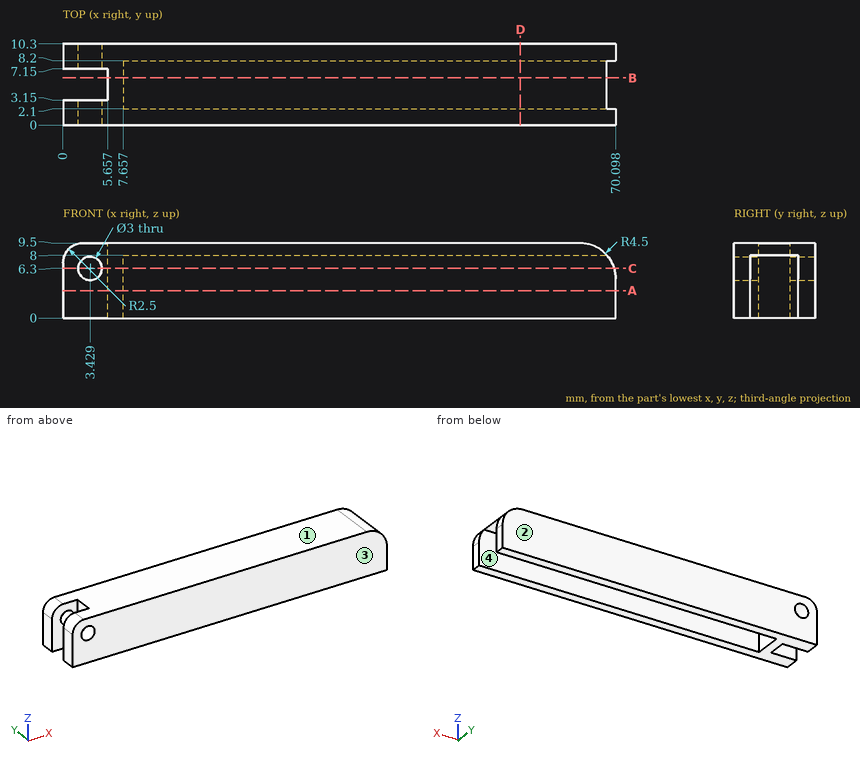
Job drawing, mm, ordinate dimensions from the low corner. One solid piece. Give positions to 0.01 mm unless a question says otherwise; leave off trailing zeros. Loops run counter-clockwise (first coordinate to the right, second up) from the corner with the lowest first, then second, coordinate; pieces in that order, holes last. Notation, with made-up numbers: M -30,32.25 L -5,32.25 A14 cw -5,58.25 Z; hole C 39,46 d1. An arc over 180 degrees is marked long. Put each result on its own line as item: value. Start each with the question number.
1) Probe probe 1 along Y at (x, z) = (52.5, 3); probe 2 along Z at (x, y) = (58, 8); probe 3 along X at (y, z) = (8, 5) (1 decimal). List the from-to ranges inside material, lowest first.
2) Saw through at A-A (z = 3.5). List the corners of the cut face in (x, y).
3) Flat gauge pins, fed straight in: pin 1 (2 mm diameter, centred on y = 5.5, z = 7, fed in from -X); pin 2 (2 mm diameter, centred on y = 6, z = 3.5, fed in from +X). Where does each tip first touch, or does it go through?
4) Pull direction Y, two halves, no side cores. Call the marked faces 1, 2, 3 and 4: +Y half, -Y half, draft (parallel to the pull), parting line (faces both ways), or undercut.
5) Saw through at D-D (x = 58). List the corners of the cut face in (y, z).
6) Saw through at B-B (y = 6). List the corners of the cut face in (x, z).
7) Saw through at C-C (z = 6.3). List the corners of the cut face in (x, y).
Numbers:
1. probe 1: 0 to 2.1, 8.2 to 10.3
1. probe 2: 8 to 9.5
1. probe 3: 0 to 2.7, 4.2 to 7.7
2. outline: M 0,0 L 70.1,0 L 70.1,2.1 L 7.66,2.1 L 7.66,8.2 L 70.1,8.2 L 70.1,10.3 L 0,10.3 L 0,7.15 L 5.66,7.15 L 5.66,3.15 L 0,3.15 Z
3. pin 1: x = 5.66
3. pin 2: x = 7.66
4. face 1: draft
4. face 2: +Y half
4. face 3: -Y half
4. face 4: undercut
5. outline: M 0,0 L 2.1,0 L 2.1,8 L 8.2,8 L 8.2,0 L 10.3,0 L 10.3,9.5 L 0,9.5 Z
6. outline: M 5.66,0 L 7.66,0 L 7.66,8 L 68.95,8 A4.5 ccw 65.6,9.5 L 5.66,9.5 Z
7. outline: M 0,0 L 1.93,0 L 1.93,3.15 L 0,3.15 Z; M 0,7.15 L 1.93,7.15 L 1.93,10.3 L 0,10.3 Z; M 4.93,0 L 69.91,0 L 69.91,2.1 L 7.66,2.1 L 7.66,8.2 L 69.91,8.2 L 69.91,10.3 L 4.93,10.3 L 4.93,7.15 L 5.66,7.15 L 5.66,3.15 L 4.93,3.15 Z
